CAD build for the part. Positions are in the model's coordinates, mm. A direction names the side the tool comes from. Coordinates: 2 decimals unless noted, no trailing zeros. Loops run counter-clockwise (first coordinate to the right, second up) from the corner with the lowest first, then second, coordinate; pieces in that order, holes last. Notation, with made-up numbers: (68, 45) -> (94, 45) arc R30 ccw to (94, 84) -> close; hole circle Ø11 at (32.25, 61.5). An arc over 180 degrees is marked (long way). Return JSON: item names as keys, results as strings. Group by question number.
(1) Flat gauge pins, fed straight in: pin 1 Ø4 at (x, y) = (-89, -48.5) entering from -Z; pin 2 Ø6 at (x, z) = (-206, 13.5) entering from +Y; pin 3 Ø6 at (y, z) = (481, 8) entering from -X. Where does each tip first touch, or does it go through?
(2) Probe L1, parallel to X at y = 562.5, z = 15.75; L2, parallel to Y at x = -154, z = 8.5; L3, parallel to Y at x = -401, z = 7.5. List the from-to ranges inside material, lowest first.
(3) Saw through at C-C on x = -437. Write the cut outline in (y, z).
(4) Saw through at A-A on z = 12.25. Write the cut outline in (x, y), then the cut area to 3 significant figures.
(5) Tool access for faces 1 (the face through (-140, 400, 10)), 2 (the face through (-102, -300, 10)): list every direction of +Z, -Z, +X, -X, +Y, -Y with a clear straight run to the whole face (end or side of a thin tool).
(6) Saw through at B-B on x = -120. Write the cut outline in (y, z), then the cut area to 3 significant figures.
```python
from build123d import *

# Parameters (mm, degrees)
BOSS_EXTRUDE1_DEPTH = 20
FILLET1_R           = 4


with BuildPart() as part:
    # Sketch1 → Boss-Extrude1 (new body)
    with BuildSketch(Plane.XY):
        with BuildLine():
            Line((-300, 400), (25, 400))
            ThreePointArc((25, 400), (32.071067812, 402.928932188), (35, 410))
            Line((35, 410), (35, 600))
            Line((35, 600), (285, 600))
            Line((285, 600), (285, 100))
            Line((285, 100), (285, -300))
            Line((285, -300), (-500, -300))
            Line((-500, -300), (-500, 200))
            ThreePointArc((-500, 200), (-441.421356237, 341.421356237), (-300, 400))
        make_face()
    extrude(amount=BOSS_EXTRUDE1_DEPTH)

    # Fillet1
    fillet1_edges = [part.edges().sort_by_distance(p)[0] for p in [
        (35, 600, 10),
    ]]
    fillet(fillet1_edges, radius=FILLET1_R)


solid = part.part
```
Geometry results:
{
 "1": {"pin 1": "z = 0", "pin 2": "y = 400", "pin 3": "x = 35"},
 "2": {"L1": "35 to 285", "L2": "-300 to 400", "L3": "-300 to 372.62"},
 "3": {"outline": "(-300, 0) -> (345.71, 0) -> (345.71, 20) -> (-300, 20) -> close"},
 "4": {"outline": "(-500, -300) -> (285, -300) -> (285, 600) -> (39, 600) arc R4 ccw to (35, 596) -> (35, 410) arc R10 cw to (25, 400) -> (-300, 400) arc R200 ccw to (-500, 200) -> close", "area": "591,000 mm²"},
 "5": {"face 1": "+Z, -Z, -X, +Y", "face 2": "+Z, -Z, +X, -X, -Y"},
 "6": {"outline": "(-300, 0) -> (400, 0) -> (400, 20) -> (-300, 20) -> close", "area": "14,000 mm²"}
}
